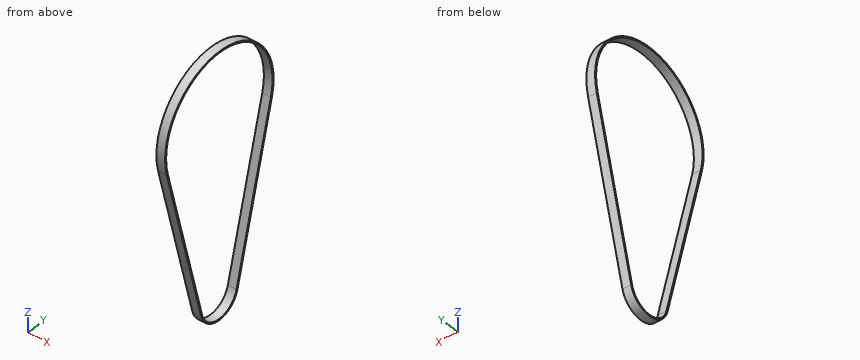
Autodesk Inventor part; units mm, degrees
ref_plane "YZ Plane" through (0, 0, 0) normal (1, 0, 0) x (0, 1, 0)
ref_plane "XZ Plane" through (0, 0, 0) normal (0, 1, 0) x (-1, 0, 0)
ref_plane "XY Plane" through (0, 0, 0) normal (0, 0, 1) x (1, 0, 0)
sketch "スケッチ1" plane through (0, 0, 0) normal (1, 0, 0) x (0, 1, 0)
  arc A0 (74.0708, -19.125) -> (-74.0708, -19.125) centre (0, 0) ccw
  arc A1 (-25.6585, -206.625) -> (25.6585, -206.625) centre (0, -200) ccw
  line L0 (74.0708, -19.125) -> (25.6585, -206.625)
  line L1 (-74.0708, -19.125) -> (-25.6585, -206.625)
  arc A2 (72.6184, -18.75) -> (-72.6184, -18.75) centre (0, 0) ccw
  arc A3 (-24.2061, -206.25) -> (24.2061, -206.25) centre (0, -200) ccw
  line L2 (-72.6184, -18.75) -> (-24.2061, -206.25)
  line L3 (72.6184, -18.75) -> (24.2061, -206.25)
  point P0 (26.5, -200)
  point P1 (-26.5, -200)
  point P2 (-26.5, -200)
  point P3 (25, -200)
  point P4 (-25, -200)
  point P5 (-62.2511, -58.9026)
  point P6 (-30.0666, -183.5524)
  dimension "d0" = 153
  dimension "d1" = 53
  dimension "d2" = 200
  dimension "d3" = 200
  dimension "d4" = 150
  dimension "d5" = 50
  dimension "d6" = 200
extrude "押し出し1" add sketch "スケッチ1" along normal blind 10
properties part number "射出_type1" material "ゴム"
Verification items for the finished model (mm, model axes). Coordinates: 2 decimals unless noted, no trailing zeros. Order: outer loops, then holes, each group sorted by start corner. A loop starts at its lowest first (then second) coordinate and runs counter-clockwise, first axis right, second up.
Item 1: Section check A-A, the plane y = 0. Enter the section's corners in (x, z), then the cut area to 3 significant figures.
Filled in:
outline: (0, -226.5) - (10, -226.5) - (10, -225) - (0, -225) - close; (0, 75) - (10, 75) - (10, 76.5) - (0, 76.5) - close
area: 30.0 mm2
Item 2: Depth check by flat-ended pin: pin 1 (3 mm diameter, centred on x = 7, y = -18.5, fed in from +Z); pin 2 (2 mm diameter, centred on x = 9, y = -24, fed in from +Z); pin 3 (1 mm diameter, centred on x = 4, y = 11.5, fed in from +Z) (3 decimals). Enter the tip coordinate at first touch or a pass-through.
Filled in:
pin 1: stops at z = 74.59
pin 2: stops at z = 72.96
pin 3: stops at z = 75.705
Item 3: Section check B-B, the plane z = 0. Enter the section's corners in (x, y).
Filled in:
outline: (0, -76.5) - (10, -76.5) - (10, -75) - (0, -75) - close; (0, 75) - (10, 75) - (10, 76.5) - (0, 76.5) - close
Item 4: Material ranges on L1, parallel to Y at x = 8, z = 0; L2, parallel to Y at x = 7.25, z = -52; L3, parallel to Z at x = 4, y = 18, recorded low to high.
Filled in:
L1: y = -76.5 to -75, 75 to 76.5
L2: y = -65.58 to -64.03, 64.03 to 65.58
L3: z = -219.45 to -217.35, 72.81 to 74.35
